```python
from build123d import *

# Parameters (mm, degrees)
SKETCH1_W                   = 120.65
SKETCH1_H                   = 76.2
BOSS_EXTRUDE1_DEPTH         = 4.7625
SKETCH2_W                   = 12.6746
SKETCH2_H                   = 4.7371
SKETCH2_W_2                 = 12.7
SKETCH2_H_2                 = 4.7625
SKETCH2_W_3                 = 12.7254
SKETCH2_H_3                 = 4.7879
SKETCH2_W_4                 = 12.7508
SKETCH2_H_4                 = 4.8133
CUT_EXTRUDE1_DEPTH          = 5.7625
F_1_4_CLEARANCE_HOLE1_D     = 6.7564
F_1_4_CLEARANCE_HOLE1_DEPTH = 25.4
F_1_4_CLEARANCE_HOLE1_TIP   = 2.029827343
SKETCH6_R                   = 1.5875
CUT_EXTRUDE2_DEPTH          = 5.7625
FILLET1_R                   = 2.54


with BuildPart() as part:
    # Sketch1 → Boss-Extrude1 (new body)
    with BuildSketch(Plane.XY):
        Rectangle(SKETCH1_W, SKETCH1_H)
    extrude(amount=BOSS_EXTRUDE1_DEPTH)

    # Sketch2 → Cut-Extrude1 (cut, through all)
    with BuildSketch(Plane.XY.offset(4.7625)):
        with Locations((-38.1, 28.575)):
            Rectangle(SKETCH2_W, SKETCH2_H)
        with Locations((12.7, 28.575)):
            Rectangle(SKETCH2_W, SKETCH2_H)
        with Locations((-38.1, 9.525)):
            Rectangle(SKETCH2_W_2, SKETCH2_H_2)
        with Locations((12.7, 9.525)):
            Rectangle(SKETCH2_W_2, SKETCH2_H_2)
        with Locations((-38.1, -9.525)):
            Rectangle(SKETCH2_W_3, SKETCH2_H_3)
        with Locations((12.7, -9.525)):
            Rectangle(SKETCH2_W_3, SKETCH2_H_3)
        with Locations((-38.1, -28.575)):
            Rectangle(SKETCH2_W_4, SKETCH2_H_4)
        with Locations((12.7, -28.575)):
            Rectangle(SKETCH2_W_4, SKETCH2_H_4)
    extrude(amount=-CUT_EXTRUDE1_DEPTH, mode=Mode.SUBTRACT)

    # 1/4 Clearance Hole1
    with Locations(Plane.XY.offset(4.7625)):
        with Locations((-50.8, 19.05), (50.8, 19.05), (-50.8, -19.05), (50.8, -19.05)):
            Hole(F_1_4_CLEARANCE_HOLE1_D / 2, depth=F_1_4_CLEARANCE_HOLE1_DEPTH)
            with Locations((0, 0, -(F_1_4_CLEARANCE_HOLE1_DEPTH + F_1_4_CLEARANCE_HOLE1_TIP / 2))):  # 118° drill point
                Cone(0, F_1_4_CLEARANCE_HOLE1_D / 2, F_1_4_CLEARANCE_HOLE1_TIP, mode=Mode.SUBTRACT)

    # Sketch6 → Cut-Extrude2 (cut, through all)
    with BuildSketch(Plane.XY.offset(4.7625)):
        with Locations((50.8, 34.925)):
            Circle(SKETCH6_R)
    extrude(amount=-CUT_EXTRUDE2_DEPTH, mode=Mode.SUBTRACT)

    # Fillet1
    fillet1_edges = [part.edges().sort_by_distance(p)[0] for p in [
        (-60.325, 38.1, 2.38125),
        (60.325, 38.1, 2.38125),
        (60.325, -38.1, 2.38125),
        (-60.325, -38.1, 2.38125),
    ]]
    fillet(fillet1_edges, radius=FILLET1_R)


solid = part.part
```
Input: part model. Units: mm. Frame: model coordinates. A direction names the side the tool comes from. Coordinates: 2 decimals unless noted, no trailing zeros. Loops run counter-clockwise (first coordinate to the right, second up) from the corner with the lowest first, then second, coordinate; pieces in that order, holes last. Notation, with made-up numbers: M -35.5,52.25 L -2.5,52.25 A15 cw -2.5,62.25 Z; hole C 53.5,56.25 d11. An arc over 180 degrees is marked long. Use a Markdown table: item, result. Add a question column.
1) Section C-C, the plane x = 50.8. Return the cut outline in (y, z).
2) Pin query (flat end, axial travel): P1, Ø4, axis at x = -50.8, y = -19.05, coming from the -Z side. Return the tip coordinate at first contact, or that it passes through.
3) Line query: L1, parallel to X at y = 26.5, z = 2.35 (3 decimals); L2, parallel to Y at x = 50.5, z = 2.15; L3, parallel to X at y = -30, z = 3.35 (3 decimals). Output: solid intervals per line, ascending. Write a range as from..to.
4) Set-up query: faces 1 (the flat face through (-44.45, 9, 2)), 2 (the flat face through (60.325, 0, 2)). Return all of +Z, -Z, +X, -X, +Y, -Y with unobstructed straight access to the full face (end or side cutting, diameter ignored); none if empty.
5) Section A-A, the plane y = -27.5. Return the cut outline in (x, z) (1 decimal), plus the area to 3 significant figures.
6) Section B-B, the plane x = -50.8. Return the cut outline in (y, z), plus the area to 3 significant figures.
7) Draft query along Y for faces 3 (the flat face through (-38, -7.131, 2)), 4 (the flat face through (-1, -38.1, 2)), 5 (the flat face through (-60.325, 0, 2)). Return one class per face: +Y half, -Y half, draft (parallel to the pull), parting line (faces both ways), or undercut.
8) Section D-D, the plane z = 2.1. Give the number of separate pieces and of enclosed holes in the cut face, plus the area to 3 significant figures.
Answer below:
| question | item | result |
|---|---|---|
| 1 | outline | M -38.1,0 L -22.43,0 L -22.43,4.76 L -38.1,4.76 Z; M -15.67,0 L 15.67,0 L 15.67,4.76 L -15.67,4.76 Z; M 22.43,0 L 33.34,0 L 33.34,4.76 L 22.43,4.76 Z; M 36.51,0 L 38.1,0 L 38.1,4.76 L 36.51,4.76 Z |
| 2 | P1 | through |
| 3 | L1 | -60.325..-44.437, -31.763..6.363, 19.037..60.325 |
| 3 | L2 | -38.1..-22.41, -15.69..15.69, 22.41..33.37, 36.48..38.1 |
| 3 | L3 | -60.325..-44.475, -31.725..6.325, 19.075..60.325 |
| 4 | face 1 | +Z, -Z |
| 4 | face 2 | +Z, -Z, +X, +Y, -Y |
| 5 | outline | M -60.3,0 L -44.5,0 L -44.5,4.8 L -60.3,4.8 Z; M -31.7,0 L 6.3,0 L 6.3,4.8 L -31.7,4.8 Z; M 19.1,0 L 60.3,0 L 60.3,4.8 L 19.1,4.8 Z |
| 5 | area | 453 mm2 |
| 6 | outline | M -38.1,0 L -22.43,0 L -22.43,4.76 L -38.1,4.76 Z; M -15.67,0 L 15.67,0 L 15.67,4.76 L -15.67,4.76 Z; M 22.43,0 L 38.1,0 L 38.1,4.76 L 22.43,4.76 Z |
| 6 | area | 299 mm2 |
| 7 | face 3 | undercut |
| 7 | face 4 | -Y half |
| 7 | face 5 | draft |
| 8 | separate pieces | 1 |
| 8 | enclosed holes | 13 |
| 8 | area | 8,550 mm2 |
